The model under review builds one solid part; all positions refer to its coordinate system, in mm. A direction names the side the tool comes from. Coordinates: 2 decimals unless noted, no trailing zeros. Write each loop counter-clockwise with the first axis right and the second up, starting at its lowest first coordinate (ties: lowest second). Pieces come first, ordered by that corner, then holes. Notation, with made-up numbers: (63.5, 48.5) - (91.5, 48.5) arc R31 cw to (91.5, 73.5) - close; hole circle Ø6 at (0.5, 73.25). An arc over 180 degrees is marked (long way). Put each result on its own line as item: value.
from build123d import *
from OCP.BRepFilletAPI import BRepFilletAPI_MakeChamfer
from build123d.topology import SkipClean

# Parameters (mm, degrees)
BOSS_EXTRUDE1_DEPTH      = 50
BOSS_EXTRUDE1_DEPTH_BACK = 10
SKETCH1_R                = 2.5
CUT_EXTRUDE1_DEPTH       = 9
CUT_EXTRUDE2_START       = -49
SKETCH3_R                = 2.5
SKETCH3_R_2              = 12.5
CUT_EXTRUDE2_DEPTH       = 49
CHAMFER1_SIZE            = 1
CHAMFER3_SIZE            = 0.25
CHAMFER3_SIZE2           = 0.184313844


with BuildPart() as part:
    # Sketch1 → Boss-Extrude1 (new, two sides: drawn at the far end of the back side and taken through both)
    with BuildSketch(Plane(origin=(0, 0, 0), x_dir=(0, 0, -1), z_dir=(1, 0, 0)).offset(-BOSS_EXTRUDE1_DEPTH_BACK)):
        with BuildLine():
            Line((-23.765647123, 13.461864934), (-13.852076656, 2.029771495))
            ThreePointArc((-13.852076656, 2.029771495), (-3.497090476, -13.556192615), (13.105341071, -4.924432496))
            Line((13.105341071, -4.924432496), (22.321723678, 19.603030839))
            ThreePointArc((22.321723678, 19.603030839), (26.290114693, 27.747382955), (25.028095201, 36.718776684))
            Line((25.028095201, 36.718776684), (14.462638657, 59.37647136))
            ThreePointArc((14.462638657, 59.37647136), (6.246574067, 67.186988673), (-5.088825774, 67.315862606))
            Line((-5.088825774, 67.315862606), (-42.598290861, 53.068728443))
            ThreePointArc((-42.598290861, 53.068728443), (-54.654931611, 23.055130592), (-23.765647123, 13.461864934))
        make_face()
        with Locations((-34.786596532, 32.502313304)):
            Circle(SKETCH1_R, mode=Mode.SUBTRACT)
        Circle(SKETCH1_R, mode=Mode.SUBTRACT)
        with Locations((10.980324502, 30.168193627)):
            Circle(SKETCH1_R, mode=Mode.SUBTRACT)
        with Locations((0.414867958, 52.825888303)):
            Circle(SKETCH1_R, mode=Mode.SUBTRACT)
        with BuildLine():
            Line((-43.786596532, 30.802313304), (-52.286596532, 30.802313304))
            ThreePointArc((-52.286596532, 30.802313304), (-53.986596532, 32.502313304), (-52.286596532, 34.202313304))
            Line((-52.286596532, 34.202313304), (-43.786596532, 34.202313304))
            ThreePointArc((-43.786596532, 34.202313304), (-42.086596532, 32.502313304), (-43.786596532, 30.802313304))
        make_face(mode=Mode.SUBTRACT)
        with BuildLine():
            Line((-40.758839718, 39.446541938), (-45.008839718, 46.80775787))
            ThreePointArc((-45.008839718, 46.80775787), (-44.386596532, 49.130001056), (-42.064353345, 48.50775787))
            Line((-42.064353345, 48.50775787), (-37.814353345, 41.146541938))
            ThreePointArc((-37.814353345, 41.146541938), (-38.436596532, 38.824298751), (-40.758839718, 39.446541938))
        make_face(mode=Mode.SUBTRACT)
        with BuildLine():
            Line((-31.758839718, 41.146541938), (-27.508839718, 48.50775787))
            ThreePointArc((-27.508839718, 48.50775787), (-25.186596532, 49.130001056), (-24.564353345, 46.80775787))
            Line((-24.564353345, 46.80775787), (-28.814353345, 39.446541938))
            ThreePointArc((-28.814353345, 39.446541938), (-31.136596532, 38.824298751), (-31.758839718, 41.146541938))
        make_face(mode=Mode.SUBTRACT)
        with BuildLine():
            Line((-25.786596532, 34.202313304), (-17.286596532, 34.202313304))
            ThreePointArc((-17.286596532, 34.202313304), (-15.586596532, 32.502313304), (-17.286596532, 30.802313304))
            Line((-17.286596532, 30.802313304), (-25.786596532, 30.802313304))
            ThreePointArc((-25.786596532, 30.802313304), (-27.486596532, 32.502313304), (-25.786596532, 34.202313304))
        make_face(mode=Mode.SUBTRACT)
        with BuildLine():
            Line((-28.814353345, 25.55808467), (-24.564353345, 18.196868737))
            ThreePointArc((-24.564353345, 18.196868737), (-25.186596532, 15.874625551), (-27.508839718, 16.496868737))
            Line((-27.508839718, 16.496868737), (-31.758839718, 23.85808467))
            ThreePointArc((-31.758839718, 23.85808467), (-31.136596532, 26.180327856), (-28.814353345, 25.55808467))
        make_face(mode=Mode.SUBTRACT)
        with BuildLine():
            Line((-37.814353345, 23.85808467), (-42.064353345, 16.496868737))
            ThreePointArc((-42.064353345, 16.496868737), (-44.386596532, 15.874625551), (-45.008839718, 18.196868737))
            Line((-45.008839718, 18.196868737), (-40.758839718, 25.55808467))
            ThreePointArc((-40.758839718, 25.55808467), (-38.436596532, 26.180327856), (-37.814353345, 23.85808467))
        make_face(mode=Mode.SUBTRACT)
    extrude(amount=BOSS_EXTRUDE1_DEPTH + BOSS_EXTRUDE1_DEPTH_BACK)

    # Sketch2 → Cut-Extrude1 (cut)
    with BuildSketch(Plane.ZY.offset(10)):
        with BuildLine():
            Line((27.472010023, 13.244670036), (10.007664514, 19.878112367))
            Line((10.007664514, 19.878112367), (12.484617032, 1.701275279))
            ThreePointArc((12.484617032, 1.701275279), (3.085967096, -12.216251761), (-11.794806964, -4.431989247))
            Line((-11.794806964, -4.431989247), (-21.420363252, 21.184403759))
            ThreePointArc((-21.420363252, 21.184403759), (-24.611724807, 28.196439271), (-23.538151999, 35.825388873))
            Line((-23.538151999, 35.825388873), (-13.270595294, 58.617284911))
            ThreePointArc((-13.270595294, 58.617284911), (-5.805096413, 65.854911183), (4.591717953, 66.007090733))
            Line((4.591717953, 66.007090733), (42.10118304, 51.759956571))
            ThreePointArc((42.10118304, 51.759956571), (54.044239799, 25.187726795), (27.472010023, 13.244670036))
        make_face()
    extrude(amount=-CUT_EXTRUDE1_DEPTH, mode=Mode.SUBTRACT)

    # Sketch3 → Cut-Extrude2 (cut)
    # profile 1 of 3: a face of its own
    with SkipClean():  # the faces are left unmerged after this step: merging them gives an invalid solid
        with BuildSketch(Plane(origin=(50, 0, 0), x_dir=(0, 0, -1), z_dir=(1, 0, 0)).offset(CUT_EXTRUDE2_START)):
            with BuildLine():
                Line((13.105341071, -4.924432496), (22.321723678, 19.603030839))
                ThreePointArc((22.321723678, 19.603030839), (1.900176918, 17.606310016), (-2.608851844, 37.623680616))
                ThreePointArc((-2.608851844, 37.623680616), (-15.031348835, 51.535777156), (-5.088825774, 67.315862606))
                Line((-5.088825774, 67.315862606), (-42.598290861, 53.068728443))
                ThreePointArc((-42.598290861, 53.068728443), (-54.654931611, 23.055130592), (-23.765647123, 13.461864934))
                Line((-23.765647123, 13.461864934), (-13.852076656, 2.029771495))
                ThreePointArc((-13.852076656, 2.029771495), (3.497090476, 13.556192615), (13.105341071, -4.924432496))
            make_face()
            with BuildLine():
                ThreePointArc((-40.758839718, 25.55808467), (-38.436596532, 26.180327856), (-37.814353345, 23.85808467))
                Line((-37.814353345, 23.85808467), (-42.064353345, 16.496868737))
                ThreePointArc((-42.064353345, 16.496868737), (-44.386596532, 15.874625551), (-45.008839718, 18.196868737))
                Line((-45.008839718, 18.196868737), (-40.758839718, 25.55808467))
            make_face(mode=Mode.SUBTRACT)
            with BuildLine():
                ThreePointArc((-31.758839718, 23.85808467), (-31.136596532, 26.180327856), (-28.814353345, 25.55808467))
                Line((-28.814353345, 25.55808467), (-24.564353345, 18.196868737))
                ThreePointArc((-24.564353345, 18.196868737), (-25.186596532, 15.874625551), (-27.508839718, 16.496868737))
                Line((-27.508839718, 16.496868737), (-31.758839718, 23.85808467))
            make_face(mode=Mode.SUBTRACT)
            with BuildLine():
                ThreePointArc((-43.786596532, 34.202313304), (-42.086596532, 32.502313304), (-43.786596532, 30.802313304))
                Line((-43.786596532, 30.802313304), (-52.286596532, 30.802313304))
                ThreePointArc((-52.286596532, 30.802313304), (-53.986596532, 32.502313304), (-52.286596532, 34.202313304))
                Line((-52.286596532, 34.202313304), (-43.786596532, 34.202313304))
            make_face(mode=Mode.SUBTRACT)
            with BuildLine():
                ThreePointArc((-37.814353345, 41.146541938), (-38.436596532, 38.824298751), (-40.758839718, 39.446541938))
                Line((-40.758839718, 39.446541938), (-45.008839718, 46.80775787))
                ThreePointArc((-45.008839718, 46.80775787), (-44.386596532, 49.130001056), (-42.064353345, 48.50775787))
                Line((-42.064353345, 48.50775787), (-37.814353345, 41.146541938))
            make_face(mode=Mode.SUBTRACT)
            with Locations((-34.786596532, 32.502313304)):
                Circle(SKETCH3_R, mode=Mode.SUBTRACT)
            with BuildLine():
                Line((-17.286596532, 30.802313304), (-25.786596532, 30.802313304))
                ThreePointArc((-25.786596532, 30.802313304), (-27.486596532, 32.502313304), (-25.786596532, 34.202313304))
                Line((-25.786596532, 34.202313304), (-17.286596532, 34.202313304))
                ThreePointArc((-17.286596532, 34.202313304), (-15.586596532, 32.502313304), (-17.286596532, 30.802313304))
            make_face(mode=Mode.SUBTRACT)
            with BuildLine():
                ThreePointArc((-27.508839718, 48.50775787), (-25.186596532, 49.130001056), (-24.564353345, 46.80775787))
                Line((-24.564353345, 46.80775787), (-28.814353345, 39.446541938))
                ThreePointArc((-28.814353345, 39.446541938), (-31.136596532, 38.824298751), (-31.758839718, 41.146541938))
                Line((-31.758839718, 41.146541938), (-27.508839718, 48.50775787))
            make_face(mode=Mode.SUBTRACT)
        # profile 2 of 3: a face of its own
        with BuildSketch(Plane(origin=(50, 0, 0), x_dir=(0, 0, -1), z_dir=(1, 0, 0)).offset(CUT_EXTRUDE2_START)):
            with BuildLine():
                ThreePointArc((11.700690218, 44.541552728), (-5.501787706, 65.514197321), (-0.493349523, 38.855378612))
                ThreePointArc((-0.493349523, 38.855378612), (17.062392728, 17.125156224), (11.700690218, 44.541552728))
            make_face()
            with Locations((0.414867958, 52.825888303)):
                Circle(SKETCH3_R, mode=Mode.SUBTRACT)
            with Locations((10.980324502, 30.168193627)):
                Circle(SKETCH3_R, mode=Mode.SUBTRACT)
        # profile 3 of 3: a face of its own
        with BuildSketch(Plane(origin=(50, 0, 0), x_dir=(0, 0, -1), z_dir=(1, 0, 0)).offset(CUT_EXTRUDE2_START)):
            Circle(SKETCH3_R_2)
            Circle(SKETCH3_R, mode=Mode.SUBTRACT)
        extrude(amount=CUT_EXTRUDE2_DEPTH, mode=Mode.SUBTRACT)

    # Chamfer1
    chamfer1_edges = [part.edges().sort_by_distance(p)[0] for p in [
        (-1, 21.877476703, 42.883839718),
        (-1, 30.802313304, 48.036596532),
        (-1, 32.502313304, 42.086596532),
        (-1, 34.202313304, 48.036596532),
        (-1, 32.502313304, 53.986596532),
        (-1, 43.127149904, 42.883839718),
        (-1, 38.824298751, 38.436596532),
        (-1, 44.827149904, 39.939353345),
        (-1, 49.130001056, 44.386596532),
        (-1, 44.827149904, 29.633839718),
        (-1, 38.824298751, 31.136596532),
        (-1, 43.127149904, 26.689353345),
        (-1, 49.130001056, 25.186596532),
        (-1, 34.202313304, 21.536596532),
        (-1, 32.502313304, 27.486596532),
        (-1, 30.802313304, 21.536596532),
        (-1, 32.502313304, 15.586596532),
        (-1, 21.877476703, 26.689353345),
        (-1, 26.180327856, 31.136596532),
        (-1, 20.177476703, 29.633839718),
        (-1, 15.874625551, 25.186596532),
        (-1, 20.177476703, 39.939353345),
        (-1, 26.180327856, 38.436596532),
        (-1, 15.874625551, 44.386596532),
    ]]
    chamfer(chamfer1_edges, length=CHAMFER1_SIZE)

    # Chamfer3: one chamfer whose edges measure the first distance from different faces: ONE call of the kernel's chamfer builder (chamfer() names one face for all edges)
    chamfer3_edges_1 = [part.edges().sort_by_distance(p)[0] for p in [
        (-1, 25.187726795, 54.044239799),
        (-1, 16.561391202, 18.739837269),
        (-1, 10.789693823, 11.246140773),
        (-1, -12.216251761, 3.085967096),
        (-1, 8.376207256, -16.607585108),
        (-1, 28.196439271, -24.611724807),
        (-1, 47.221336892, -18.404373646),
        (-1, 65.854911183, -5.805096413),
        (-1, 58.883523652, 23.346450497),
    ]]
    chamfer3_edges_2 = [part.edges().sort_by_distance(p)[0] for p in [
        (-5.5, 19.878112367, 10.007664514),
    ]]
    chamfer3_side_2 = [part.faces().sort_by_distance(p)[0] for p in [
        (-5.5, 10.789693823, 11.246140773),
    ]]
    chamfer3 = BRepFilletAPI_MakeChamfer(part.part.solid().wrapped)
    for e in chamfer3_edges_1:
        chamfer3.Add(CHAMFER3_SIZE, e.wrapped)
    for e in chamfer3_edges_2:
        chamfer3.Add(CHAMFER3_SIZE, CHAMFER3_SIZE2, e.wrapped, chamfer3_side_2[0].wrapped)  # the first distance lies on this face
    add(Compound.cast(chamfer3.Shape()), mode=Mode.REPLACE)


solid = part.part
1. Consider section C-C on z = -18.5. State the section outline as (x, y) points, plus the area to 3 significant figures.
Determined:
outline: (-10, 9.43) - (1, 9.43) - (1, 16.61) - (50, 16.61) - (50, 17.9) - (1, 17.9) - (1, 42.44) - (50, 42.44) - (50, 50.72) - (-10, 50.72) - (-10, 47.01) - (-1.25, 47.01) - (-1, 46.4) - (-1, 14.12) - (-1.25, 13.41) - (-10, 13.41) - close
area: 621 mm^2
2. The part is to be moulded in two halves that separate along Y. For faces 4 (the flat face through (-4.58, 7.83, 18.88)), 5 (the flat face through (19.58, 47.89, -19.82)), 6 (the flat face through (-0.507, 22.079, 43.353)), say which applies: +Y half, -Y half, draft (parallel to the pull), parting line (faces both ways), or undercut.
Determined:
face 4: -Y half
face 5: +Y half
face 6: undercut
3. Consider section A-A on x = 44. State the section outline as (y, z) points, plus the area to 3 significant figures.
Determined:
outline: circle Ø28 at (0, 0); (36.72, -25.03) - (59.38, -14.46) arc R15.5 ccw (long way) to (37.62, 2.61) arc R15.5 ccw (long way) to start; hole circle Ø25 at (0, 0); hole (38.86, 0.49) arc R14.39 ccw (long way) to (44.54, -11.7) arc R14 ccw (long way) to start
area: 371 mm^2
4. For pin 1 Ø3 at (y, z) = (33.5, 20.5) entering from -X; pin 2 Ø8 at (x, y) = (23, 52.5) entering from +Z; pin 3 Ø17 at (y, z) = (52.83, -0.41) entering from -X, all flat-tipped, find the tip position at first contact; note any pin that passes through.
Determined:
pin 1: stops at x = -0.8
pin 2: stops at z = 15.09
pin 3: stops at x = -1
5. Consider section B-B on y = 0. State the section outline as (x, z) points, plus the area to 3 significant figures.
Determined:
outline: (-10, -14.96) - (1, -14.96) - (1, -14) - (50, -14) - (50, -12.5) - (1, -12.5) - (1, -2.5) - (-1, -2.5) - (-1, -13.19) - (-1.25, -13.46) - (-10, -13.46) - close; (-10, 12.6) - (-1.25, 12.6) - (-1, 12.35) - (-1, 2.5) - (1, 2.5) - (1, 12.5) - (50, 12.5) - (50, 14) - (-10, 14) - close
area: 221 mm^2
6. To check wall thickness, follow probe 1 along Y at (x, z) = (0, 0); probe 2 along X at (y, z) = (30, -7); probe 3 along Y at (x, z) = (23, -1.5). State the ranges of each line that lie inside material, in increasing order.
Determined:
probe 1: y = -14 to -2.5, 2.5 to 50.36, 55.29 to 68.32
probe 2: x = -1 to 1
probe 3: y = -13.92 to -12.41, 12.41 to 13.92, 17.91 to 19.34, 66.78 to 68.29
7. Machinability: for faces 1 (the flat face through (0.49, 20.23, 39.91)), 2 (the flat face through (1, 42, -6)), 3 (the flat face through (-5.7, 16.5, 18.9)), which of the approach directions +Z, -Z, +X, -X, +Y, -Y give a long, thin tool a straight path to every point of the face, cutting with its end or side? Answer none if there is none.
Determined:
face 1: +X, -X
face 2: +X
face 3: -X
